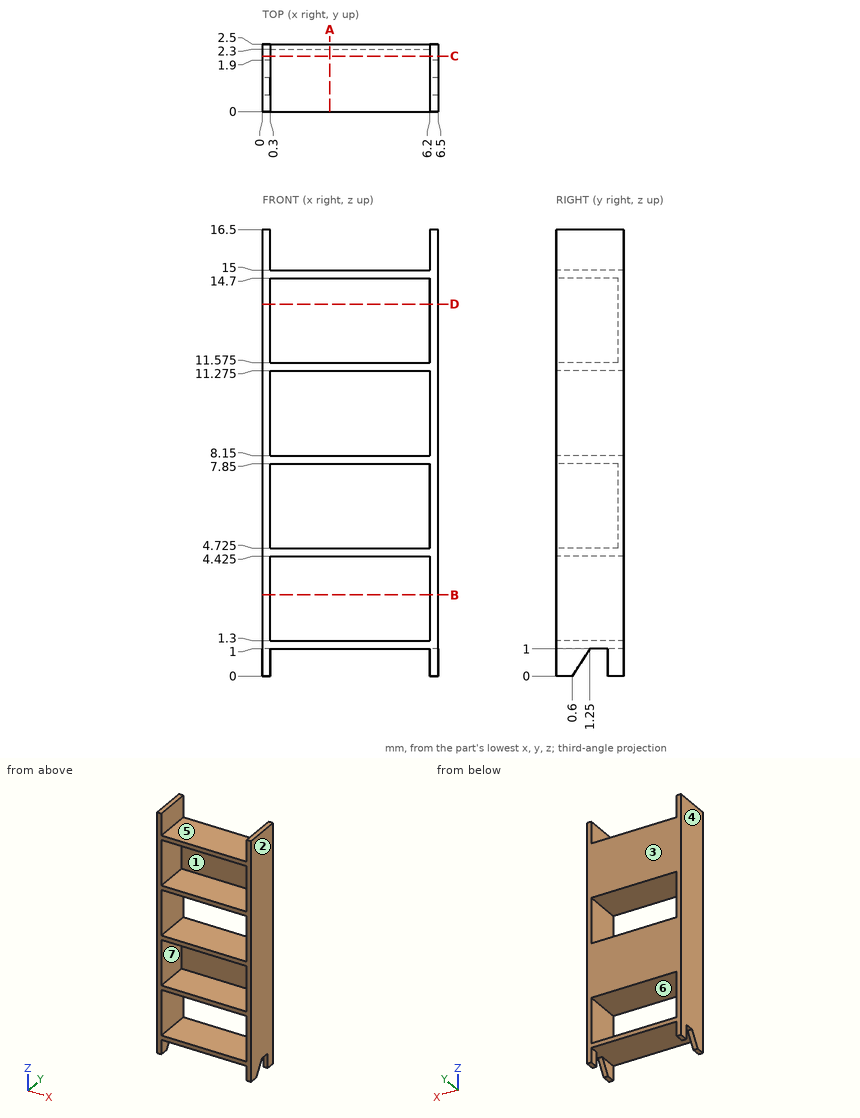
Here's the drawing with two shaded views (mm, measured from the low corner). I have some questions. A direction names the side the tool comes from. Give positions to 0.01 mm unless a question says otherwise; leave off trailing zeros. Loops run counter-clockwise (first coordinate to the right, second up) from the corner with the lowest first, then second, coordinate; pieces in that order, holes last. Notation, with made-up numbers: M 41.5,87.5 L 70.5,87.5 A17 cw 70.5,119.5 Z; hole C 73,-26.75 d9. An arc over 180 degrees is marked long. Use one line per item in the form item = value. Start each with the question number.
(1) Please list where these lines run through material, in increasing order: line 1 (Z direction, x = 3.75, y = 2.25) (3 decimals); line 2 (X direction, y = 0.2, z = 13.5); line 3 (Y direction, x = 5.25, z = 12).
(2) I'm going to push a flat-ended pin straight in: P1, Ø0.7, axis at x = 3.5, y = 1, coming from the -Z side. Where does the tip first touch, or does it pass through?
(3) Thinking about a two-plate mould opening in X: for the marked faces 1, 2 and 3, which applies, released by +X, released by -X, zero draft, split by the parting line, or undercut?
(4) I want a section at B-B, the plane z = 3. Write out the boundary of the cut face in (x, y).
(5) I want a section at A-A, the plane x = 2.5. Write out the boundary of the cut face in (y, z) (3 decimals), and give its area (3 significant figures).
(6) On a 3-axis mill with a long thin cutter (end or side, diameter ignored), from which of +Z, -Z, +X, -X, +Y, -Y can I reach the whole of each face in a straight line? I mean the marked faces 4, 5, 6 and 7. Say none if no direction works.
(7) I want a section at C-C, the plane y = 2.05. Write out the boundary of the cut face in (x, z) (3 decimals).
(8) I want a section at D-D, the plane z = 13.75. Write out the boundary of the cut face in (x, y), and give its area (3 significant figures).
Worked out:
q1.line_1 = 1 to 1.3, 4.425 to 4.725, 7.85 to 8.15, 11.275 to 11.575, 14.7 to 15
q1.line_2 = 0 to 0.3, 6.2 to 6.5
q1.line_3 = 2.3 to 2.5
q2.P1 = 1
q3.face_1 = undercut
q3.face_2 = released by +X
q3.face_3 = zero draft
q4.outline = M 0,0 L 0.3,0 L 0.3,2.5 L 0,2.5 Z; M 6.2,0 L 6.5,0 L 6.5,2.5 L 6.2,2.5 Z
q5.outline = M 0,1 L 2.5,1 L 2.5,1.3 L 0,1.3 Z; M 0,4.425 L 2.5,4.425 L 2.5,8.15 L 0,8.15 L 0,7.85 L 2.3,7.85 L 2.3,4.725 L 0,4.725 Z; M 0,11.275 L 2.5,11.275 L 2.5,15 L 0,15 L 0,14.7 L 2.3,14.7 L 2.3,11.575 L 0,11.575 Z
q5.area = 5.00 mm²
q6.face_4 = +Z, -Z, -X, +Y, -Y
q6.face_5 = +Z, +Y, -Y
q6.face_6 = +Y, -Y
q6.face_7 = -Y
q7.outline = M 0,0 L 0.3,0 L 0.3,1 L 6.2,1 L 6.2,0 L 6.5,0 L 6.5,16.5 L 6.2,16.5 L 6.2,15 L 0.3,15 L 0.3,16.5 L 0,16.5 Z; hole M 0.3,1.3 L 6.2,1.3 L 6.2,4.425 L 0.3,4.425 Z; hole M 0.3,4.725 L 6.2,4.725 L 6.2,7.85 L 0.3,7.85 Z; hole M 0.3,8.15 L 6.2,8.15 L 6.2,11.275 L 0.3,11.275 Z; hole M 0.3,11.575 L 6.2,11.575 L 6.2,14.7 L 0.3,14.7 Z
q8.outline = M 0,0 L 0.3,0 L 0.3,2.3 L 6.2,2.3 L 6.2,0 L 6.5,0 L 6.5,2.5 L 0,2.5 Z
q8.area = 2.68 mm²
